```python
from build123d import *

# Parameters (mm, degrees)
SKETCH1_R           = 8.999999998
BOSS_EXTRUDE1_DEPTH = 20
SKETCH2_R           = 14.270327874
BOSS_EXTRUDE2_DEPTH = 5
SKETCH3_R           = 6.549662412
CUT_EXTRUDE1_DEPTH  = 18


with BuildPart() as part:
    # Sketch1 → Boss-Extrude1 (new body)
    with BuildSketch(Plane(origin=(0, 0, 1384.443253532), x_dir=(-1, 0, 0), z_dir=(0, 0, -1))):
        with Locations(Location((-588.451811663, 952.777089149, 0), (0, 0, 90))):
            Circle(SKETCH1_R)
    extrude(amount=-BOSS_EXTRUDE1_DEPTH)

    # Sketch2 → Boss-Extrude2 (add)
    with BuildSketch(Plane(origin=(0, 0, 1384.443253532), x_dir=(-1, 0, 0), z_dir=(0, 0, -1))):
        with Locations(Location((-588.451811663, 952.777089149, 0), (0, 0, 90))):
            Circle(SKETCH2_R)
    extrude(amount=BOSS_EXTRUDE2_DEPTH)

    # Sketch3 → Cut-Extrude1 (cut)
    with BuildSketch(Plane.XY.offset(1404.443253532)):
        with Locations((588.451811663, 952.777089149)):
            Circle(SKETCH3_R)
    extrude(amount=-CUT_EXTRUDE1_DEPTH, mode=Mode.SUBTRACT)


solid = part.part
```
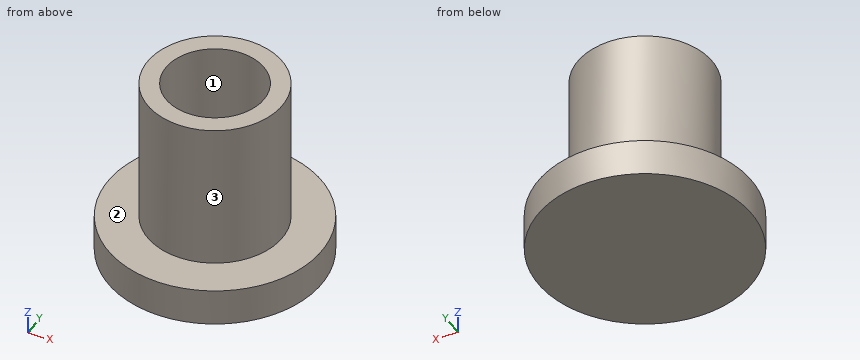
CAD build for the part. Positions are in the model's coordinates, mm. Face numbers are marked on the shaded views. Give positions to 0.01 mm unless a question says otherwise; leave off trailing zeros. Loops run counter-clockwise (first coordinate to the right, second up) from the corner with the lowest first, then second, coordinate; pieces in that order, holes last. Notation, with made-up numbers: M -9,50 L 3,50 A21 cw 3,62 Z; hole C -13.5,22.25 d11. An arc over 180 degrees is marked long. Use one line per item in the form item = value.
Item 1: Drill centre lines: probe 1 along Y at (x, z) = (588.75, 1392.75); probe 2 along X at (y, z) = (953, 1401.75); probe 3 along Z at (x, y) = (584, 962.5). Where is each one in solid material? Low to high. Write a range as from..to.
Determined:
probe_1 = 943.78..946.23, 959.32..961.77
probe_2 = 579.45..581.91, 595..597.45
probe_3 = 1379.44..1384.44
Item 2: Slice it at D-D (x = 590). List the corners of the cut face in (y, z).
Determined:
outline = M 938.59,1379.44 L 966.96,1379.44 L 966.96,1384.44 L 961.64,1384.44 L 961.64,1404.44 L 959.14,1404.44 L 959.14,1386.44 L 946.41,1386.44 L 946.41,1404.44 L 943.91,1404.44 L 943.91,1384.44 L 938.59,1384.44 Z
Item 3: Slice it at A-A (y = 960). List the corners of the cut face in (x, z).
Determined:
outline = M 576.14,1379.44 L 600.76,1379.44 L 600.76,1384.44 L 593.82,1384.44 L 593.82,1404.44 L 583.08,1404.44 L 583.08,1384.44 L 576.14,1384.44 Z
Item 4: Two-plate mould, pull along Y, no slides. Class the marked faces 1, 2 and 3: pulls with the +Y half, pulls with the -Y half, needs draft (parallel to the pull), parting line crosses it, or undercut.
Determined:
face_1 = undercut
face_2 = needs draft
face_3 = parting line crosses it
Item 5: Slice it at B-B (x = 580.25). List the corners of the cut face in (y, z).
Determined:
outline = M 941.1,1379.44 L 964.45,1379.44 L 964.45,1384.44 L 956.48,1384.44 L 956.48,1404.44 L 949.07,1404.44 L 949.07,1384.44 L 941.1,1384.44 Z
Item 6: Flat gauge pins, fed straight in: pin 1 (4 mm diameter, centred on x = 590.5, z = 1398.5, fed in from +Y); pin 2 (6.5 mm diameter, centred on x = 590, y = 955, fed in from +Z); pin 3 (17 mm diameter, centred on x = 588.45, y = 952.78, fed in from +Z); pin 4 (12 mm diameter, centred on x = 599, z = 1398.5, fed in from +Y). Where does each tip first touch, or does it go through?
Determined:
pin_1 = 961.78
pin_2 = 1386.44
pin_3 = 1404.44
pin_4 = 960.54
Item 7: Slice it at C-C (z = 1399.5). List the corners of the cut face in (x, y).
Determined:
outline = C 588.45,952.78 d18; hole C 588.45,952.78 d13.1
